from build123d import *

# Parameters (mm, degrees)
EXTRUDE_1_DEPTH = 19
CHAMFER_1_SIZE  = 1


with BuildPart() as part:
    # 草图1 → 凸台-拉伸1 (new body)
    with BuildSketch(Plane(origin=(0, 0, 0), x_dir=(1, 0, 0), z_dir=(0, 1, 0))):
        with BuildLine():
            Line((60, -225.142177301), (60, -205))
            Line((60, -205), (85, -205))
            Line((85, -205), (85, -221.768460336))
            ThreePointArc((85, -221.768460336), (0, -237.5), (-85, -221.768460336))
            Line((-85, -221.768460336), (-85, -205))
            Line((-85, -205), (-60, -205))
            Line((-60, -205), (-60, -225.142177301))
            ThreePointArc((-60, -225.142177301), (0, -233), (60, -225.142177301))
        make_face()
    extrude(amount=EXTRUDE_1_DEPTH)

    # 倒角1
    chamfer_1_edges = [part.edges().sort_by_distance(p)[0] for p in [
        (-72.5, 0, 205),
        (-72.5, 19, 205),
        (60, 9.5, 205),
        (85, 9.5, 205),
        (-85, 9.5, 205),
        (-60, 9.5, 205),
        (72.5, 19, 205),
        (72.5, 0, 205),
    ]]
    chamfer(chamfer_1_edges, length=CHAMFER_1_SIZE)


solid = part.part
Can you work these out from the model? Positions are in its coordinate system, mm. A direction names the side the tool comes from. Round coordinates to 2 decimals unless told otherwise and drop trailing zeros. Loops run counter-clockwise (first coordinate to the right, second up) from the corner with the lowest first, then second, coordinate; pieces in that order, holes last. Notation, with made-up numbers: (20.5, -32.5) - (43.5, -32.5) arc R18 ccw to (43.5, -16.5) - close; hole circle Ø4 at (41, 82). An arc over 180 degrees is marked (long way). Write item = value, one per line. Start each with the question number.
(1) If we section it at A-A (z = 210.5): Please give me the cut outline in (x, y).
(2) If we section it at C-C (x = -72.5): Please give me the cut outline in (y, z), and give its area (3 significant figures).
(3) If we mould it in two halves opening along X, with no side actions, what happens to faces 1 (the face through (-85, 9, 214)), 2 (the face through (-60, 9, 215)), 3 (the face through (1.217, 9.367, 237.497))? For each: released by +X, released by -X, zero draft, split by the parting line, or undercut.
(4) If I drill on probe 1 along X at (y, z) = (17, 211); probe 2 along Z at (x, y) = (18, 7.75); probe 3 along Z at (x, y) = (-50, 13.25), over which ranges is the centre line in solid material (lowest first)? Write a range as [from, to].
(5) For faces 4 (the face through (60, 9, 216)), 5 (the face through (0, 0, 235)), which set-ups out of +Z, -Z, +X, -X, +Y, -Y let a thin tool reach every point of the face, with its end or its side?
(6) For P1, Ø3, axis at x = 25, y = 14, coming from the +Z side; P2, Ø3, axis at x = 58.5, y = 16.5, coming from the +Z side; P3, Ø1.5, axis at x = 21, y = 7, coming from the -Z side, each with a flat end and sliding along its axis, tell me the tip position at first contact or that it passes through.
(7) If we section it at D-D (z = 227.5): Please give me the cut outline in (x, y).
(8) If we section it at B-B (y = 7.5): Please give me the cut outline in (x, z), and give its area (3 significant figures).
Ans:
q1.outline = (-85, 0) - (-60, 0) - (-60, 19) - (-85, 19) - close; (60, 0) - (85, 0) - (85, 19) - (60, 19) - close
q2.outline = (0, 206) - (1, 205) - (18, 205) - (19, 206) - (19, 226.16) - (0, 226.16) - close
q2.area = 401 mm²
q3.face_1 = released by -X
q3.face_2 = undercut
q3.face_3 = split by the parting line
q4.probe_1 = [-85, -60], [60, 85]
q4.probe_2 = [232.3, 236.82]
q4.probe_3 = [227.57, 232.18]
q5.face_4 = -Z, +Y, -Y
q5.face_5 = +Z, -Z, +X, -X, -Y
q6.P1 = 236.33
q6.P2 = 230.56
q6.P3 = 231.98
q7.outline = (-68.19, 0) - (-50.33, 0) - (-50.33, 19) - (-68.19, 19) - close; (50.33, 0) - (68.19, 0) - (68.19, 19) - (50.33, 19) - close
q8.outline = (-85, 206) - (-84, 205) - (-61, 205) - (-60, 206) - (-60, 225.14) arc R233 cw to (60, 225.14) - (60, 206) - (61, 205) - (84, 205) - (85, 206) - (85, 221.77) arc R237.5 ccw to (-85, 221.77) - close
q8.area = 1,600 mm²
